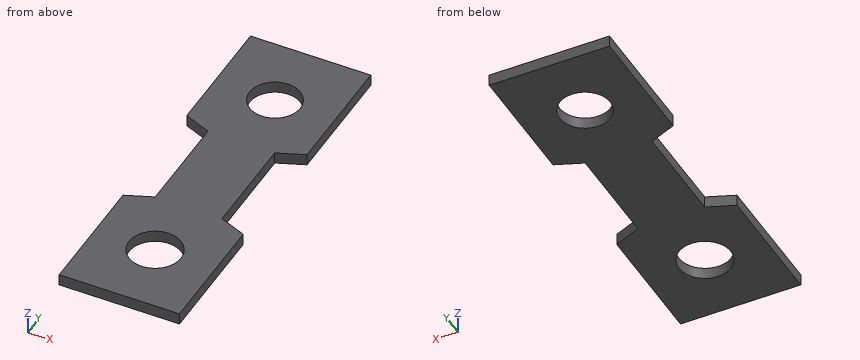
from build123d import *

# Parameters (mm, degrees)
SKETCH1_R           = 2.430870735
SKETCH1_R_2         = 2.36295848
BOSS_EXTRUDE1_DEPTH = 1.0922


with BuildPart() as part:
    # Sketch1 → Boss-Extrude1 (new body)
    with BuildSketch(Plane.XY):
        Polygon((-5.6261, 28.5115), (5.6261, 28.5115), (5.6261, 16.8275), (3.1242, 15.8115), (3.1242, 6.1595), (5.6261, 5.1435), (5.6261, -6.5405), (-5.6261, -6.5405), (-5.6261, 5.1435), (-3.1242, 6.1595), (-3.1242, 15.8115), (-5.6261, 16.8275), align=None)
        Circle(SKETCH1_R, mode=Mode.SUBTRACT)
        with Locations((0, 21.971)):
            Circle(SKETCH1_R_2, mode=Mode.SUBTRACT)
    extrude(amount=BOSS_EXTRUDE1_DEPTH)


solid = part.part
Work out the finished part from the listing and answer in its coordinate system (mm). Round coordinates to 2 decimals unless told otherwise and drop trailing zeros. Loops run counter-clockwise (first coordinate to the right, second up) from the corner with the lowest first, then second, coordinate; pieces in that order, holes last. Notation, with made-up numbers: (31.5, 47.5) - (40.5, 47.5) arc R6 ccw to (40.5, 58.5) - close; hole circle Ø9 at (23, -5). An arc over 180 degrees is marked (long way). One line per item, written item: value.
Q1. Straight lines are drawn through the part: probe 1 along Y at (x, z) = (0, 0.9); probe 2 along Y at (x, z) = (1.75, 0.4); probe 3 along X at (y, z) = (22, 0.4). For each, find the intervals that lie inside material, in ascending order.
Check values:
probe 1: -6.54 to -2.43, 2.43 to 19.61, 24.33 to 28.51
probe 2: -6.54 to -1.69, 1.69 to 20.38, 23.56 to 28.51
probe 3: -5.63 to -2.36, 2.36 to 5.63
Q2. Find section B-B on x = 0. Give the vertices of the cut face in (y, z), and give its area (3 significant figures).
Check values:
outline: (-6.54, 0) - (-2.43, 0) - (-2.43, 1.09) - (-6.54, 1.09) - close; (2.43, 0) - (19.61, 0) - (19.61, 1.09) - (2.43, 1.09) - close; (24.33, 0) - (28.51, 0) - (28.51, 1.09) - (24.33, 1.09) - close
area: 27.8 mm2
Q3. Find section C-C on z = 0.2. Give the vertices of the cut face in (x, y), and give its area (3 significant figures).
Check values:
outline: (-5.63, -6.54) - (5.63, -6.54) - (5.63, 5.14) - (3.12, 6.16) - (3.12, 15.81) - (5.63, 16.83) - (5.63, 28.51) - (-5.63, 28.51) - (-5.63, 16.83) - (-3.12, 15.81) - (-3.12, 6.16) - (-5.63, 5.14) - close; hole circle Ø4.86 at (0, 0); hole circle Ø4.73 at (0, 21.97)
area: 305 mm2
Q4. Each of these flat-tipped pins is pushed along its axis until it touches: pin 1 Ø3 at (x, y) = (0, 0) entering from +Z; pin 2 Ø2 at (x, y) = (1.5, 23) entering from +Z. Where does it stop, or does it pass through?
Check values:
pin 1: through
pin 2: z = 1.09
Q5. Find section D-D on x = -3.5. Give the vertices of the cut face in (y, z).
Check values:
outline: (-6.54, 0) - (6.01, 0) - (6.01, 1.09) - (-6.54, 1.09) - close; (15.96, 0) - (28.51, 0) - (28.51, 1.09) - (15.96, 1.09) - close
Q6. Find section A-A on y = 0. Give the vertices of the cut face in (x, z).
Check values:
outline: (-5.63, 0) - (-2.43, 0) - (-2.43, 1.09) - (-5.63, 1.09) - close; (2.43, 0) - (5.63, 0) - (5.63, 1.09) - (2.43, 1.09) - close
